Work out the finished part from the listing and answer in its coordinate system (mm). Face numbers are marked on the shaded views. A direction names the side the tool comes from. Round coordinates to 2 decimals unless told otherwise and drop trailing zeros. Write each loop counter-clockwise with the first axis right and the second up, starting at its lowest first coordinate (ties: lowest second). Pieces come first, ordered by that corner, then holes.
1. Determine the mould class of the marked faces 3, 4 and 5 for opening direction Y: pulls with the +Y half, pulls with the -Y half, needs draft (parallel to the pull), parting line crosses it, or undercut.
2. Find section B-B (x = 0). Write down the section's boundary in (y, z).
3. Find section A-A (y = 0). Write down the section's boundary in (x, z), and give its area (3 significant figures).
4. A tool of negligible diameter and unlimited length cuts with its end or side. For the marked faces 1 and 2, from which of +Z, -Z, +X, -X, +Y, -Y can it reach the whole face along a straight path? Write none if from no direction.
5. Flat-ended cylindrical pins translate along their axes: pin 1 Ø4 at (x, z) = (-7, 19.5) entering from -Y; pin 2 Ø1 at (y, z) = (18.5, 8.5) entering from -X; pin 3 Ø1 at (x, z) = (18, 15.5) entering from +Y. Find the tip coordinate at first contact, or state that the pin passes through.
6. Straight lines are drawn through the part: probe 1 along Y at (x, z) = (0, 8); probe 2 along Y at (x, z) = (-3.5, 11.5); probe 3 along Z at (x, y) = (13.5, 0). For each, find the intervals that lie inside material, in ascending order.
7. Find section D-D (y = -9.5). Write down the section's boundary in (x, z).
8. Find section C-C (z = 7.5). Write down the section's boundary in (x, y), and give its area (3 significant figures).
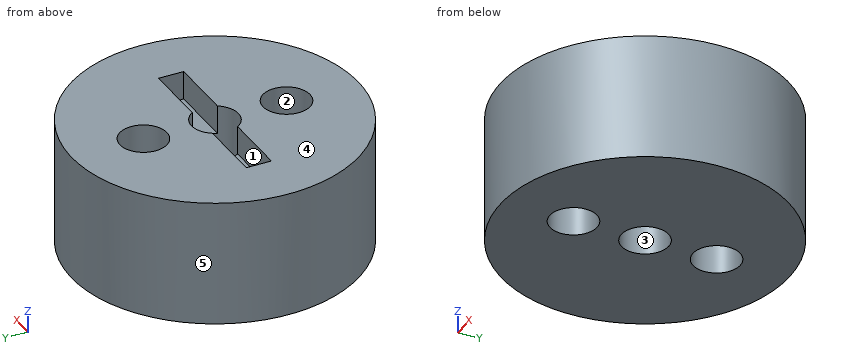
```python
from build123d import *

# Parameters (mm, degrees)
F0_R     = 25
F0_R_2   = 4.1
F1_DEPTH = 22
F2_W     = 30
F2_H     = 4.4
F3_DEPTH = 5


with BuildPart() as f1:
    # F0 (on Top) → F1 (new body)
    with BuildSketch(Plane.XY):
        Circle(F0_R)
        with Locations((0, -12.5)):
            Circle(F0_R_2, mode=Mode.SUBTRACT)
        Circle(F0_R_2, mode=Mode.SUBTRACT)
        with Locations((0, 12.5)):
            Circle(F0_R_2, mode=Mode.SUBTRACT)
    extrude(amount=F1_DEPTH)

    # F2 (on face) → F3 (cut)
    with BuildSketch(Plane.XY.offset(22)):
        Rectangle(F2_W, F2_H)
    extrude(amount=-F3_DEPTH, mode=Mode.SUBTRACT)


solid = f1.part
```
Worked answers:
1. face 3: undercut
1. face 4: needs draft
1. face 5: parting line crosses it
2. outline: (-25, 0) - (-16.6, 0) - (-16.6, 22) - (-25, 22) - close; (-8.4, 0) - (-4.1, 0) - (-4.1, 22) - (-8.4, 22) - close; (4.1, 0) - (8.4, 0) - (8.4, 22) - (4.1, 22) - close; (16.6, 0) - (25, 0) - (25, 22) - (16.6, 22) - close
3. outline: (-25, 0) - (-4.1, 0) - (-4.1, 17) - (-15, 17) - (-15, 22) - (-25, 22) - close; (4.1, 0) - (25, 0) - (25, 22) - (15, 22) - (15, 17) - (4.1, 17) - close
3. area: 811 mm2
4. face 1: +Z
4. face 2: +Z, -Z
5. pin 1: stops at y = -24.49
5. pin 2: stops at x = -17.35
5. pin 3: stops at y = 17.85
6. probe 1: y = -25 to -16.6, -8.4 to -4.1, 4.1 to 8.4, 16.6 to 25
6. probe 2: y = -24.75 to -14.64, -10.36 to -2.14, 2.14 to 10.36, 14.64 to 24.75
6. probe 3: z = 0 to 17
7. outline: (-23.12, 0) - (-2.79, 0) - (-2.79, 22) - (-23.12, 22) - close; (2.79, 0) - (23.12, 0) - (23.12, 22) - (2.79, 22) - close
8. outline: circle Ø50 at (0, 0); hole circle Ø8.2 at (0, -12.5); hole circle Ø8.2 at (0, 0); hole circle Ø8.2 at (0, 12.5)
8. area: 1,810 mm2
